from build123d import *
from build123d.topology import SkipClean

# Parameters (mm, degrees)
BOSS_EXTRUDE1_DEPTH             = 12.7
F_19_0_166_DIAMETER_HOLE1_D     = 4.2164
F_19_0_166_DIAMETER_HOLE1_DEPTH = 15.875
F_19_0_166_DIAMETER_HOLE1_TIP   = 1.266734357


# Read off the part's stored shape, not the designer's step: #8-32 Tapped Hole1
with BuildPart() as part:
    # Sketch1 → Boss-Extrude1 (new body)
    with BuildSketch(Plane.XY):
        with BuildLine():
            Line((9.525, -77.909402237), (9.525, -86.8045))
            ThreePointArc((9.525, -86.8045), (9.376210245, -87.163710245), (9.017, -87.3125))
            Line((9.017, -87.3125), (-9.017, -87.3125))
            ThreePointArc((-9.017, -87.3125), (-9.376210245, -87.163710245), (-9.525, -86.8045))
            Line((-9.525, -86.8045), (-9.525, -77.909402237))
            ThreePointArc((-9.525, -77.909402237), (-9.145773261, -77.059049719), (-8.259734198, -76.77296039))
            ThreePointArc((-8.259734198, -76.77296039), (0, -77.216), (8.259734198, -76.77296039))
            ThreePointArc((8.259734198, -76.77296039), (9.145773261, -77.059049719), (9.525, -77.909402237))
        make_face()
    extrude(amount=BOSS_EXTRUDE1_DEPTH)

    # #19 (0.166) Diameter Hole1
    with Locations(Plane.XY.offset(12.7)):
        with Locations((4.7752, -82.55), (-4.7752, -82.55)):
            Hole(F_19_0_166_DIAMETER_HOLE1_D / 2, depth=F_19_0_166_DIAMETER_HOLE1_DEPTH)
            with Locations((0, 0, -(F_19_0_166_DIAMETER_HOLE1_DEPTH + F_19_0_166_DIAMETER_HOLE1_TIP / 2))):  # 118° drill point
                Cone(0, F_19_0_166_DIAMETER_HOLE1_D / 2, F_19_0_166_DIAMETER_HOLE1_TIP, mode=Mode.SUBTRACT)

    # #8-32 Tapped Hole1 outline → #8-32 Tapped Hole1 (revolve, cut)
    with SkipClean():  # the faces are left unmerged after this step: merging them gives an invalid solid
        with BuildSketch(Plane.XY.offset(7.9502)):
            Polygon((2.54, -77.216), (2.54, -77.174195215), (0, -77.174194503), (0, -87.3125), (2.286, -87.3125), (1.7272, -86.7537), (1.7272, -78.0288), align=None)
        revolve(axis=Axis((0, 0, 7.9502), (0, 1, 0)), mode=Mode.SUBTRACT)


solid = part.part
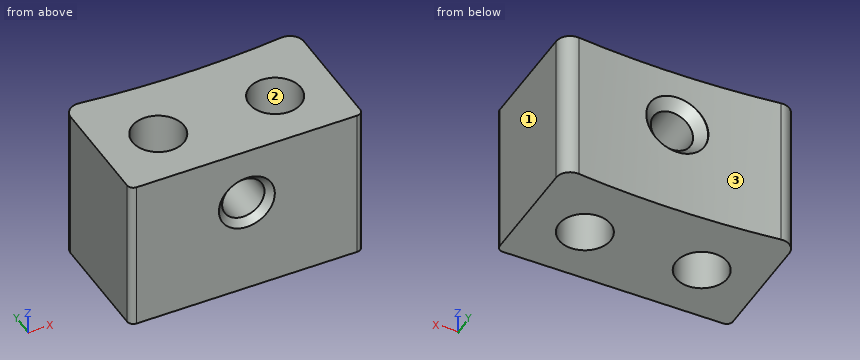
Here's how the part is built. I have some questions about the finished solid (model axes, mm). Face numbers are marked on the shaded views. Coordinates: 2 decimals unless noted, no trailing zeros. Write each loop counter-clockwise with the first axis right and the second up, starting at its lowest first coordinate (ties: lowest second). Pieces come first, ordered by that corner, then holes. Notation, with made-up numbers: (-1, 72) - (57, 72) arc R22 ccw to (57, 90) - close; hole circle Ø7 at (-24.75, -5). An arc over 180 degrees is marked (long way). Use one line per item in the form item = value.
1) Suppose I cut it at D-D, the plane y = -83.75. Write out the boundary of the cut face in (x, z) (3 decimals), plus the area to 3 significant figures.
Solved:
outline = (-9.525, 0) - (-6.509, 0) - (-6.509, 12.7) - (-9.525, 12.7) - close; (-3.042, 0) - (3.042, 0) - (3.042, 12.7) - (-3.042, 12.7) - close; (6.509, 0) - (9.525, 0) - (9.525, 12.7) - (6.509, 12.7) - close; hole circle Ø3.454 at (0, 7.95)
area = 145 mm2
2) Suppose I cut it at B-B, the plane y = -82.55. Write out the boundary of the cut face in (x, z) (3 decimals).
Solved:
outline = (-9.525, 0) - (-6.883, 0) - (-6.883, 12.7) - (-9.525, 12.7) - close; (-2.667, 0) - (2.667, 0) - (2.667, 12.7) - (-2.667, 12.7) - close; (6.883, 0) - (9.525, 0) - (9.525, 12.7) - (6.883, 12.7) - close; hole circle Ø3.454 at (0, 7.95)
3) Thinking about a two-plate mould opening in Y: for the marked faces 1, 2 and 3, which applies, released by +Y, released by -Y, zero draft, split by the parting line, or undercut?
Solved:
face_1 = zero draft
face_2 = undercut
face_3 = released by +Y
4) I need wall thicknesses on line 1 (X direction, y = -86.5, z = 8) (3 decimals); line 2 (X direction, y = -83.5, z = 4) (3 decimals); line 3 (Z direction, x = 0, y = -84.25). Which ranges of each line are inside material? Lowest first, please.
Solved:
line_1 = -9.525 to -1.726, 1.726 to 9.525
line_2 = -9.525 to -6.657, -2.893 to 2.893, 6.657 to 9.525
line_3 = 0 to 6.22, 9.68 to 12.7
5) Suppose I cut it at A-A, the plane z = 1.5. Give the number of separate pieces and of enclosed holes in the cut face, plus the area to 3 significant figures.
Solved:
separate_pieces = 1
enclosed_holes = 2
area = 167 mm2
6) Suppose I cut it at C-C, the plane x = -4. Write out the boundary of the cut face in (y, z).
Solved:
outline = (-87.31, 0) - (-84.51, 0) - (-84.51, 12.7) - (-87.31, 12.7) - close; (-80.59, 0) - (-77.11, 0) - (-77.11, 12.7) - (-80.59, 12.7) - close
